```python
from build123d import *

# Parameters (mm, degrees)
BOSS_EXTRUDE2_DEPTH = 50.8


with BuildPart() as part:
    # Sketch1 → Boss-Extrude2 (new body)
    with BuildSketch(Plane.XY):
        with BuildLine():
            Line((0, 48.477635603), (0, 889))
            ThreePointArc((0, 889), (7.439487758, 906.960512242), (25.4, 914.4))
            Line((25.4, 914.4), (1239.487859684, 914.4))
            ThreePointArc((1239.487859684, 914.4), (1263.732503571, 896.573456464), (1253.945793147, 868.116318332))
            Line((1253.945793147, 868.116318332), (39.857933462, 27.593953935))
            ThreePointArc((39.857933462, 27.593953935), (13.611690324, 25.978841081), (0, 48.477635603))
        make_face()
        with BuildLine():
            Line((120.072727273, 180.3859565), (120.072727273, 841.663636364))
            ThreePointArc((120.072727273, 841.663636364), (123.792471152, 850.643892485), (132.772727273, 854.363636364))
            Line((132.772727273, 854.363636364), (227.445454545, 854.363636364))
            ThreePointArc((227.445454545, 854.363636364), (236.425710667, 850.643892485), (240.145454545, 841.663636364))
            Line((240.145454545, 841.663636364), (240.145454545, 245.928613843))
            ThreePointArc((240.145454545, 245.928613843), (238.694851807, 240.034459004), (234.674421277, 235.486773009))
            Line((234.674421277, 235.486773009), (140.001694004, 169.944115666))
            ThreePointArc((140.001694004, 169.944115666), (126.878572434, 169.136559239), (120.072727273, 180.3859565))
        make_face(mode=Mode.SUBTRACT)
        with BuildLine():
            Line((360.218181818, 346.640501955), (360.218181818, 841.663636364))
            ThreePointArc((360.218181818, 841.663636364), (363.937925697, 850.643892485), (372.918181818, 854.363636364))
            Line((372.918181818, 854.363636364), (467.590909091, 854.363636364))
            ThreePointArc((467.590909091, 854.363636364), (476.571165212, 850.643892485), (480.290909091, 841.663636364))
            Line((480.290909091, 841.663636364), (480.290909091, 412.183159297))
            ThreePointArc((480.290909091, 412.183159297), (478.840306352, 406.289004459), (474.819875822, 401.741318463))
            Line((474.819875822, 401.741318463), (380.147148549, 336.198661121))
            ThreePointArc((380.147148549, 336.198661121), (367.02402698, 335.391104693), (360.218181818, 346.640501955))
        make_face(mode=Mode.SUBTRACT)
        with BuildLine():
            Line((600.363636364, 512.895047409), (600.363636364, 841.663636364))
            ThreePointArc((600.363636364, 841.663636364), (604.083380243, 850.643892485), (613.063636364, 854.363636364))
            Line((613.063636364, 854.363636364), (707.736363636, 854.363636364))
            ThreePointArc((707.736363636, 854.363636364), (716.716619757, 850.643892485), (720.436363636, 841.663636364))
            Line((720.436363636, 841.663636364), (720.436363636, 578.437704752))
            ThreePointArc((720.436363636, 578.437704752), (718.985760898, 572.543549914), (714.965330368, 567.995863918))
            Line((714.965330368, 567.995863918), (620.292603095, 502.453206575))
            ThreePointArc((620.292603095, 502.453206575), (607.169481525, 501.645650148), (600.363636364, 512.895047409))
        make_face(mode=Mode.SUBTRACT)
        with BuildLine():
            Line((840.509090909, 679.149592864), (840.509090909, 841.663636364))
            ThreePointArc((840.509090909, 841.663636364), (844.228834788, 850.643892485), (853.209090909, 854.363636364))
            Line((853.209090909, 854.363636364), (1087.951598187, 854.363636364))
            ThreePointArc((1087.951598187, 854.363636364), (1100.07392013, 845.450364596), (1095.180564918, 831.22179553))
            Line((1095.180564918, 831.22179553), (860.43805764, 668.70775203))
            ThreePointArc((860.43805764, 668.70775203), (847.314936071, 667.900195602), (840.509090909, 679.149592864))
        make_face(mode=Mode.SUBTRACT)
    extrude(amount=BOSS_EXTRUDE2_DEPTH)


solid = part.part
```
Read the model definition and answer for the solid it produces. Units are mm, in the model's axes. A direction names the side the tool comes from. Give positions to 0.01 mm unless a question says otherwise; leave off trailing zeros. Write each loop counter-clockwise with the first axis right and the second up, starting at its lowest first coordinate (ties: lowest second). Pieces come first, ordered by that corner, then holes. Notation, with made-up numbers: (-4.75, -0.75) -> (40.25, -0.75) arc R32 cw to (40.25, 36.25) -> close; hole circle Ø10 at (-30, 79.5). An arc over 180 degrees is marked (long way). Answer in a Markdown table with one row per item.
1) A tool of negligible diameter and unlimited length cuts with its end or side. For faces 1 (the flat face through (120.073, 506, 25)), 2 (the cylindrical face through (7.24, 906.76, 25.04)), from which of +Z, -Z, +X, -X, +Y, -Y can it reach the whole face along a straight path? Write none if from no direction.
Results list:
| item | result |
|---|---|
| face 1 | +Z, -Z |
| face 2 | +Z, -Z, -X, +Y |
2) Section C-C on z = 33.5 is taken. Count the separate pieces of the cut face and the enclosed holes in it, plus the area to 3 significant figures.
Results list:
| item | result |
|---|---|
| separate pieces | 1 |
| enclosed holes | 4 |
| area | 398,000 mm^2 |
3) Straight lines are drawn through the part: line 1 (X direction, y = 429.5, z = 11); line 2 (Y direction, x = 667.5, z = 19); line 3 (Y direction, x = 433, z = 44.5). For each, find the intervals that lie inside material, in ascending order. Write a range as [from, to].
Results list:
| item | result |
|---|---|
| line 1 | [0, 120.07], [240.15, 360.22], [480.29, 620.39] |
| line 2 | [462.12, 535.14], [854.36, 914.4] |
| line 3 | [299.77, 372.79], [854.36, 914.4] |
4) Each of these flat-tipped pins is pushed along its axis until it touches: pin 1 Ø5 at (x, z) = (358.5, 44.5) entering from -Y; pin 2 Ø3 at (x, z) = (545, 16) entering from -Y; pin 3 Ø5 at (y, z) = (593, 33) entering from +X. Where does it stop, or does it pass through?
Results list:
| item | result |
|---|---|
| pin 1 | y = 246.46 |
| pin 2 | y = 376.27 |
| pin 3 | x = 860.17 |
5) Section A-A on x = 978.5 is taken. Give the vertices of the cut face in (y, z), plus the area to 3 significant figures.
Results list:
| item | result |
|---|---|
| outline | (677.42, 0) -> (750.44, 0) -> (750.44, 50.8) -> (677.42, 50.8) -> close; (854.36, 0) -> (914.4, 0) -> (914.4, 50.8) -> (854.36, 50.8) -> close |
| area | 6,760 mm^2 |
6) Determine the mould class of faces 3 (the flat face through (655.4, 453.74, 25.04)), 4 (the flat face through (240.145, 548, 25)), 5 (the flat face through (624, 914.4, 25)) for opening direction X: released by +X, released by -X, zero draft, split by the parting line, or undercut.
Results list:
| item | result |
|---|---|
| face 3 | released by +X |
| face 4 | undercut |
| face 5 | zero draft |
7) Section B-B on y = 271 is taken. Give the vertices of the cut face in (x, z).
Results list:
| item | result |
|---|---|
| outline | (0, 0) -> (120.07, 0) -> (120.07, 50.8) -> (0, 50.8) -> close; (240.15, 0) -> (391.44, 0) -> (391.44, 50.8) -> (240.15, 50.8) -> close |
8) Section D-D on y = 647 is taken. Give the vertices of the cut face in (x, z).
Results list:
| item | result |
|---|---|
| outline | (0, 0) -> (120.07, 0) -> (120.07, 50.8) -> (0, 50.8) -> close; (240.15, 0) -> (360.22, 0) -> (360.22, 50.8) -> (240.15, 50.8) -> close; (480.29, 0) -> (600.36, 0) -> (600.36, 50.8) -> (480.29, 50.8) -> close; (720.44, 0) -> (934.56, 0) -> (934.56, 50.8) -> (720.44, 50.8) -> close |
